```python
from build123d import *

# Parameters (mm, degrees)
F0_W     = 152.4
F0_H     = 231.775
F0_W_2   = 25.4
F0_W_3   = 76.2
F1_DEPTH = 4.7625
F2_W     = 4.7625
F2_H     = 231.775
F3_DEPTH = 25.4
F4_W     = 4.7625
F4_H     = 9.525
F5_DEPTH = 9.525


with BuildPart() as f1:
    # F0 (on Top) → F1 (new body)
    with BuildSketch(Plane.XY):
        Rectangle(F0_W, F0_H)
        with Locations((-88.9, 0)):
            Rectangle(F0_W_2, F0_H)
        with Locations((-139.7, 0)):
            Rectangle(F0_W_3, F0_H)
    extrude(amount=F1_DEPTH)

    # F2 (on face) → F3 (join)
    with BuildSketch(Plane.XY.offset(4.7625)):
        with Locations((-175.41875, 0)):
            Rectangle(F2_W, F2_H)
    extrude(amount=F3_DEPTH)

    # F4 (on face) → F5 (join)
    with BuildSketch(Plane(origin=(0, 0, 0), x_dir=(1, 0, 0), z_dir=(0, 0, -1))):
        with Locations((67.46875, 73.025)):
            Rectangle(F4_W, F4_H)
        with Locations((67.46875, -73.025)):
            Rectangle(F4_W, F4_H)
        with Locations((67.46875, 82.55)):
            Rectangle(F4_W, F4_H)
        with Locations((67.46875, -82.55)):
            Rectangle(F4_W, F4_H)
    extrude(amount=-F5_DEPTH)


solid = f1.part
```
The model under review builds one solid part; all positions refer to its coordinate system, in mm. Give positions to 0.01 mm unless a question says otherwise; leave off trailing zeros. Write each loop counter-clockwise with the first axis right and the second up, starting at its lowest first coordinate (ties: lowest second). Pieces come first, ordered by that corner, then holes.
(1) For P1, Ø1.5, axis at x = -136.5, y = -90.5, coming from the +Z side; P2, Ø5, axis at x = 68, z = 6.5, coming from the -Y side; P3, Ø1, axis at y = -72, z = 26.5, coming from the +X side; P4, Ø4, axis at x = 67.5, z = 7, coming from the +Y side, all flat-tipped, find the tip position at first contact; note any pin that passes through.
(2) Consider section C-C, the plane z = 16. Give the boundary of the cut face in (x, y), and give its area (3 significant figures).
(3) Consider section A-A, the plane x = 13.5. Give the boundary of the cut face in (y, z), and give its area (3 significant figures).
(4) To check wall thickness, follow L1, parallel to X at y = -31.5, z = 5.5; L2, parallel to Z at x = -113, y = 10.5. State the ranges of each line that lie inside material, in increasing order.
(5) Consider section B-B, the plane y = -32. Give the boundary of the cut face in (x, z).
Returned:
1. P1: stops at z = 4.76
1. P2: stops at y = -115.89
1. P3: stops at x = -173.04
1. P4: stops at y = 87.31
2. outline: (-177.8, -115.89) - (-173.04, -115.89) - (-173.04, 115.89) - (-177.8, 115.89) - close
2. area: 1,100 mm2
3. outline: (-115.89, 0) - (115.89, 0) - (115.89, 4.76) - (-115.89, 4.76) - close
3. area: 1,100 mm2
4. L1: x = -177.8 to -173.04
4. L2: z = 0 to 4.76
5. outline: (-177.8, 0) - (76.2, 0) - (76.2, 4.76) - (-173.04, 4.76) - (-173.04, 30.16) - (-177.8, 30.16) - close
